Check sheet for the drawn part. Datum: minimum x, y, z corner. Units: mm. Give positions to 0.01 mm unless a question says otherwise; leave off trailing zeros. Loops run counter-clockwise (first coordinate to the right, second up) from the corner with the lowest first, then second, coordinate; pieces in that order, holes last.
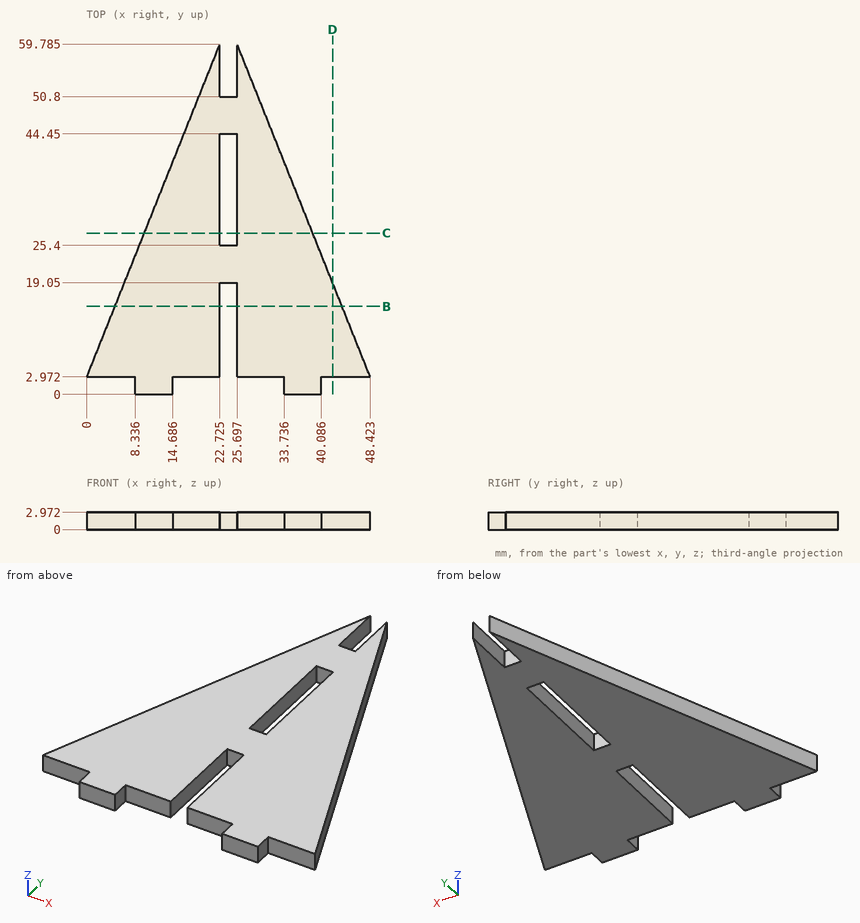
(1) Gauge pin test, flat ends, axial feed: pin 1 Ø0.9 at (y, z) = (14.5, 1) entering from +X; pin 2 Ø8 at (x, y) = (9, 43.5) entering from +Z; pin 3 Ø1.5 at (x, z) = (25, 1.5) entering from +Y (1 decimal); pin 4 Ø1.5 at (y, z) = (57.5, 1) entering from +X. Record the tip position at first contact, or that the pin passes through.
(2) Material ranges on line 1 (X direction, y = 4.5, z = 0.85) (1 decimal); line 2 (X direction, y = 40, z = 1.05) (1 decimal); line 3 (Y direction, x = 3.5, z = 2.5) (1 decimal), recorded low to high.
(3) Section check C-C on y = 27.5. Record the boundary of the cut face in (x, z) (1 decimal).
(4) Section check D-D on x = 42. Record the boundary of the cut face in (y, z).
(5) Section check B-B on y = 15. Record the boundary of the cut face in (x, z) (1 decimal).
Computed values:
1. pin 1: stops at x = 43.99
1. pin 2: passes through
1. pin 3: stops at y = 59.8
1. pin 4: stops at x = 26.91
2. line 1: x = 0.6 to 22.7, 25.7 to 47.8
2. line 2: x = 14.8 to 22.7, 25.7 to 33.6
2. line 3: y = 3 to 11.7
3. outline: (9.8, 0) - (22.7, 0) - (22.7, 3) - (9.8, 3) - close; (25.7, 0) - (38.6, 0) - (38.6, 3) - (25.7, 3) - close
4. outline: (2.97, 0) - (19.03, 0) - (19.03, 2.97) - (2.97, 2.97) - close
5. outline: (4.8, 0) - (22.7, 0) - (22.7, 3) - (4.8, 3) - close; (25.7, 0) - (43.6, 0) - (43.6, 3) - (25.7, 3) - close
